CAD build for the part. Positions are in the model's coordinates, mm. Face numbers are marked on the shaded views. A direction names the side the tool comes from. Give positions to 0.01 mm unless a question says otherwise; leave off trailing zeros. Write each loop counter-clockwise with the first axis right and the second up, starting at its lowest first coordinate (ties: lowest second). Pieces come first, ordered by that corner, then holes. Notation, with made-up numbers: (77.5, -25) - (105.5, -25) arc R23 ccw to (105.5, 0) - close; hole circle Ø4 at (75, 34.5). An arc over 180 degrees is marked (long way). Answer as a JSON object with one key per item and string values.
Autodesk Inventor part; units mm, degrees
ref_plane "YZ Plane" through (0, 0, 0) normal (1, 0, 0) x (0, 1, 0)
ref_plane "XZ Plane" through (0, 0, 0) normal (0, 1, 0) x (-1, 0, 0)
ref_plane "XY Plane" through (0, 0, 0) normal (0, 0, 1) x (1, 0, 0)
sketch "Эскиз1" plane through (0, 0, 0) normal (0, 1, 0) x (-1, 0, 0)
  line L0 (-50, 50) -> (50, 50)
  line L1 (50, 50) -> (50, -50)
  line L2 (50, -50) -> (-50, -50)
  line L3 (-50, -50) -> (-50, 50)
  line L4 (-50, 50) -> (50, -50) construction
  line L5 (50, 50) -> (-50, -50) construction
  point P0 (0, 0)
  dimension "d0" = 100
  dimension "d1" = 100
extrude "Выдавливание1" add sketch "Эскиз1" along normal mid plane 100
sketch "Эскиз2" plane through (-50, 50, 50) normal (0, 0, 1) x (1, 0, 0)
  circle A0 centre (50, -50) radius 35
  dimension "d4" = 70
extrude "Выдавливание2" add sketch "Эскиз2" along normal blind 10
properties part number "motor" material "Пластик АБС"
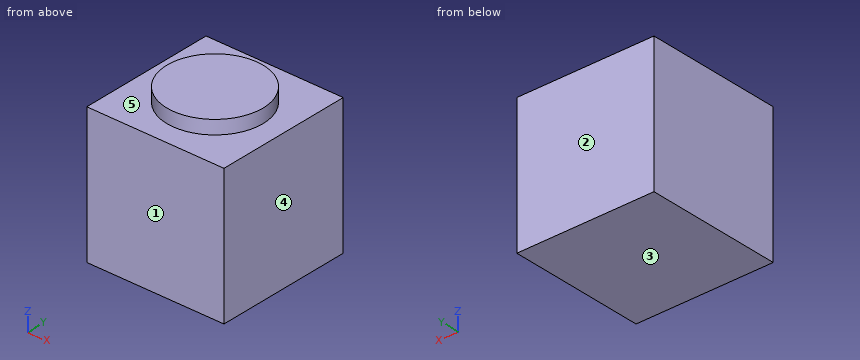
Item 1: Which spindle directions (+Z, -Z, +X, -X, +Y, -Y) get a long thin tool onto all of the face, cutting with end or side? Do the marked faces 4 and 5. Say none if no direction does.
Entries:
{"face 4": "+Z, -Z, +X, +Y, -Y", "face 5": "+Z"}
Item 2: Probe line 1 (Z direction, x = -38, y = 29); line 2 (X direction, y = -21, z = 54.5). List the from-to ranges inside material, lowest first. Write a range as from..to.
Entries:
{"line 1": "-50..50", "line 2": "-28..28"}
Item 3: Cut at A-A (y = 0). Give the cut face in (x, z), and give its area (3 significant figures).
Entries:
{"outline": "(-50, -50) - (50, -50) - (50, 50) - (35, 50) - (35, 60) - (-35, 60) - (-35, 50) - (-50, 50) - close", "area": "10,700 mm2"}
Item 4: Mould opens along Y. For the marked faces 1, 2 and 3 say: +Y half, -Y half, draft (parallel to the pull), parting line (faces both ways), or undercut.
Entries:
{"face 1": "-Y half", "face 2": "+Y half", "face 3": "draft"}
Item 5: Cut at C-C (x = 42). Give the cut face in (y, z).
Entries:
{"outline": "(-50, -50) - (50, -50) - (50, 50) - (-50, 50) - close"}
